```python
from build123d import *

# Parameters (mm, degrees)
SKETCH1_W           = 283
SKETCH1_H           = 225
BOSS_EXTRUDE1_DEPTH = 80.2
SKETCH2_W           = 258
SKETCH2_H           = 200
CUT_EXTRUDE1_DEPTH  = 80.2
SKETCH3_W           = 10
SKETCH3_H           = 10
BOSS_EXTRUDE2_DEPTH = 60.16
SKETCH4_R           = 5
BOSS_EXTRUDE3_DEPTH = 10


with BuildPart() as part:
    # Sketch1 → Boss-Extrude1 (new body)
    with BuildSketch(Plane(origin=(0, 0, 0), x_dir=(1, 0, 0), z_dir=(0, 1, 0))):
        with Locations((141.5, 112.5)):
            Rectangle(SKETCH1_W, SKETCH1_H)
    extrude(amount=BOSS_EXTRUDE1_DEPTH)

    # Sketch2 → Cut-Extrude1 (cut)
    with BuildSketch(Plane(origin=(0, 80.2, 0), x_dir=(1, 0, 0), z_dir=(0, 1, 0))):
        with Locations((141.5, 112.5)):
            Rectangle(SKETCH2_W, SKETCH2_H)
    extrude(amount=-CUT_EXTRUDE1_DEPTH, mode=Mode.SUBTRACT)

    # Sketch3 → Boss-Extrude2 (add)
    with BuildSketch(Plane.XZ):
        with Locations((17.5, -17.5)):
            Rectangle(SKETCH3_W, SKETCH3_H)
        with Locations((17.5, -207.5)):
            Rectangle(SKETCH3_W, SKETCH3_H)
        with Locations((265.5, -207.5)):
            Rectangle(SKETCH3_W, SKETCH3_H)
        with Locations((265.5, -17.5)):
            Rectangle(SKETCH3_W, SKETCH3_H)
    extrude(amount=-BOSS_EXTRUDE2_DEPTH)

    # Sketch4 → Boss-Extrude3 (add)
    with BuildSketch(Plane.XZ):
        with Locations(Location((17.5, -17.5, 0), (0, 0, 270))):
            Circle(SKETCH4_R)
        with Locations(Location((265.5, -17.5, 0), (0, 0, 270))):
            Circle(SKETCH4_R)
        with Locations(Location((265.5, -207.5, 0), (0, 0, 90))):
            Circle(SKETCH4_R)
        with Locations(Location((17.5, -207.5, 0), (0, 0, 90))):
            Circle(SKETCH4_R)
    extrude(amount=BOSS_EXTRUDE3_DEPTH)


solid = part.part
```
Check sheet for the modelled part. Datum: model origin and axes. Units: mm. A direction names the side the tool comes from. Round coordinates to 2 decimals unless told otherwise and drop trailing zeros. Order: outer loops, then holes, each group sorted by start corner. A loop starts at its lowest first (then second) coordinate and runs counter-clockwise, first axis right, second up. Notation, with made-up numbers: M 77,41 L 134,41 A18 cw 134,72 Z; hole C -5,-1 d3. An arc over 180 degrees is marked long. Answer in a Markdown table with one row per item.
(1) Section check B-B on x = 143. Record the boundary of the cut face in (y, z), plus the area to 4 significant figures.
Findings:
| item | result |
|---|---|
| outline | M 0,-225 L 80.2,-225 L 80.2,-212.5 L 0,-212.5 Z; M 0,-12.5 L 80.2,-12.5 L 80.2,0 L 0,0 Z |
| area | 2,005 mm^2 |
(2) Material ranges on line 1 along Z through (x, y) = (116.5, 2); line 2 along X through (y, z) = (10, -87); line 3 along X through (y, z) = (27, -20), recorded low to high. Write a range as from..to.
Findings:
| item | result |
|---|---|
| line 1 | z = -225..-212.5, -12.5..0 |
| line 2 | x = 0..12.5, 270.5..283 |
| line 3 | x = 0..22.5, 260.5..283 |
(3) Gauge pin test, flat end, axial feed: pin 1 (11 mm diameter, centred on x = 263.5, z = -205.5, fed in from +Y). Record the tip position at first contact, or that the pin passes through.
Findings:
| item | result |
|---|---|
| pin 1 | stops at y = 60.16 |
(4) Section check A-A on z = -138.5. Record the boundary of the cut face in (x, y), plus the area to 4 significant figures.
Findings:
| item | result |
|---|---|
| outline | M 0,0 L 12.5,0 L 12.5,80.2 L 0,80.2 Z; M 270.5,0 L 283,0 L 283,80.2 L 270.5,80.2 Z |
| area | 2,005 mm^2 |
(5) Section check C-C on y = 15. Record the boundary of the cut face in (x, z).
Findings:
| item | result |
|---|---|
| outline | M 0,-225 L 283,-225 L 283,0 L 0,0 Z; hole M 12.5,-202.5 L 22.5,-202.5 L 22.5,-212.5 L 260.5,-212.5 L 260.5,-202.5 L 270.5,-202.5 L 270.5,-22.5 L 260.5,-22.5 L 260.5,-12.5 L 22.5,-12.5 L 22.5,-22.5 L 12.5,-22.5 Z |
(6) Set-up check for faces 5 (the flat face through (17, 30, -22.5)), 6 (the flat face through (140, 40, -225)), 7 (the cylindrical face through (16, -4.93, -202.73)), 8 (the flat face through (265, 60.16, -17)), 9 (the flat face through (283, 40, -111)): record each of +Z, -Z, +X, -X, +Y, -Y from which the full face is reachable in a straight line by a thin tool's end or side.
Findings:
| item | result |
|---|---|
| face 5 | +Y, -Y |
| face 6 | -Z, +X, -X, +Y, -Y |
| face 7 | -Y |
| face 8 | +Y |
| face 9 | +Z, -Z, +X, +Y, -Y |
(7) Draft check along X on faces 1 (the flat face through (260.5, 30, -208)), 2 (the flat face through (0, 40, -111)), 3 (the flat face through (265, -10, -208)), 4 (the flat face through (12.5, 41, -111)). Enter one of: +X half, -X half, draft (parallel to the pull), parting line (faces both ways), or undercut.
Findings:
| item | result |
|---|---|
| face 1 | undercut |
| face 2 | -X half |
| face 3 | draft |
| face 4 | undercut |
